```python
from build123d import *

# Parameters (mm, degrees)
SKETCH1_W           = 50.8
SKETCH1_H           = 67.8
SKETCH1_R           = 2.58125
SKETCH1_R_2         = 12.7
SKETCH1_R_3         = 2.613
BOSS_EXTRUDE1_DEPTH = 3.175
CHAMFER1_SIZE       = 3.175


with BuildPart() as part:
    # Sketch1 → Boss-Extrude1 (new body)
    with BuildSketch(Plane.XY):
        with Locations((-25.4, 33.9)):
            Rectangle(SKETCH1_W, SKETCH1_H)
        with Locations((-38.1, 12.7)):
            Circle(SKETCH1_R, mode=Mode.SUBTRACT)
        with Locations(Location((-12.7, 12.7, 0), (0, 0, 180))):
            Circle(SKETCH1_R, mode=Mode.SUBTRACT)
        with Locations((-25.4, 46.8)):
            Circle(SKETCH1_R_2, mode=Mode.SUBTRACT)
        with Locations((-42.9, 64.3)):
            Circle(SKETCH1_R_3, mode=Mode.SUBTRACT)
        with Locations(Location((-7.9, 64.3, 0), (0, 0, 180))):
            Circle(SKETCH1_R_3, mode=Mode.SUBTRACT)
        with Locations((-7.9, 29.3)):
            Circle(SKETCH1_R_3, mode=Mode.SUBTRACT)
        with Locations(Location((-42.9, 29.3, 0), (0, 0, 180))):
            Circle(SKETCH1_R_3, mode=Mode.SUBTRACT)
    extrude(amount=BOSS_EXTRUDE1_DEPTH)

    # Chamfer1
    chamfer1_edges = [part.edges().sort_by_distance(p)[0] for p in [
        (-50.8, 67.8, 1.5875),
        (0, 67.8, 1.5875),
    ]]
    chamfer(chamfer1_edges, length=CHAMFER1_SIZE)


solid = part.part
```
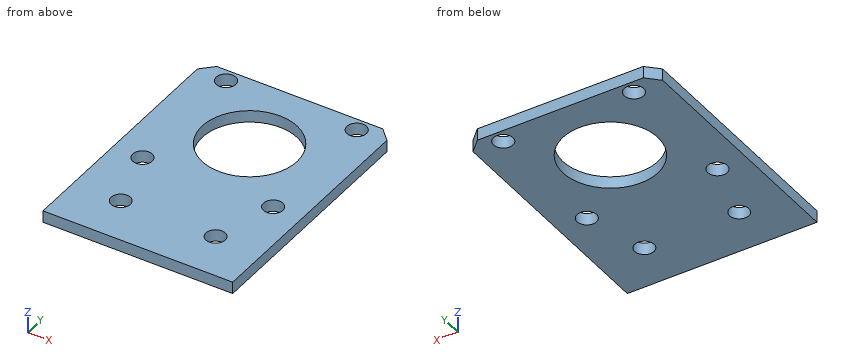
Design review of the part built by this model. Coordinates are the model's own, in mm. Coordinates: 2 decimals unless noted, no trailing zeros. Order: outer loops, then holes, each group sorted by start corner. A loop starts at its lowest first (then second) coordinate and runs counter-clockwise, first axis right, second up.
1) Wall thickness on line 1 along Y through (x, z) = (-7.9, 1.9); line 2 along Y through (x, z) = (-37, 2.7); line 3 along Y through (x, z) = (-12.5, 3): over which ranges is each line inside the solid? List them lowest first.
2) Take a section at A-A, the plane y = 12.7. Give the boundary of the cut face in (x, z) (3 decimals).
3) Take a section at C-C, the plane x = -42.9. Give the boundary of the cut face in (y, z) (3 decimals), and give its area (3 significant figures).
4) Take a section at D-D, the plane z = 1.4. Give the boundary of the cut face in (x, y) (1 decimal).
5) Take a section at B-B, the plane x = -25.4. Give the boundary of the cut face in (y, z) (3 decimals).
6) Clearance check with a flat-ended pin moving along its axis: pin 1 (23 mm diameter, centred on x = -25.4, y = 46.8, fed in from +Z). State where the tip first meets the part, or that it passes through.
Returned:
1. line 1: y = 0 to 26.69, 31.91 to 61.69, 66.91 to 67.8
1. line 2: y = 0 to 10.36, 15.04 to 41.63, 51.97 to 67.8
1. line 3: y = 0 to 10.13, 15.27 to 67.8
2. outline: (-50.8, 0) - (-40.681, 0) - (-40.681, 3.175) - (-50.8, 3.175) - close; (-35.519, 0) - (-15.281, 0) - (-15.281, 3.175) - (-35.519, 3.175) - close; (-10.119, 0) - (0, 0) - (0, 3.175) - (-10.119, 3.175) - close
3. outline: (0, 0) - (26.687, 0) - (26.687, 3.175) - (0, 3.175) - close; (31.913, 0) - (61.687, 0) - (61.687, 3.175) - (31.913, 3.175) - close; (66.913, 0) - (67.8, 0) - (67.8, 3.175) - (66.913, 3.175) - close
3. area: 182 mm2
4. outline: (-50.8, 0) - (0, 0) - (0, 64.6) - (-3.2, 67.8) - (-47.6, 67.8) - (-50.8, 64.6) - close; hole circle Ø5.2 at (-42.9, 29.3); hole circle Ø5.2 at (-42.9, 64.3); hole circle Ø5.2 at (-38.1, 12.7); hole circle Ø25.4 at (-25.4, 46.8); hole circle Ø5.2 at (-12.7, 12.7); hole circle Ø5.2 at (-7.9, 29.3); hole circle Ø5.2 at (-7.9, 64.3)
5. outline: (0, 0) - (34.1, 0) - (34.1, 3.175) - (0, 3.175) - close; (59.5, 0) - (67.8, 0) - (67.8, 3.175) - (59.5, 3.175) - close
6. pin 1: passes through
